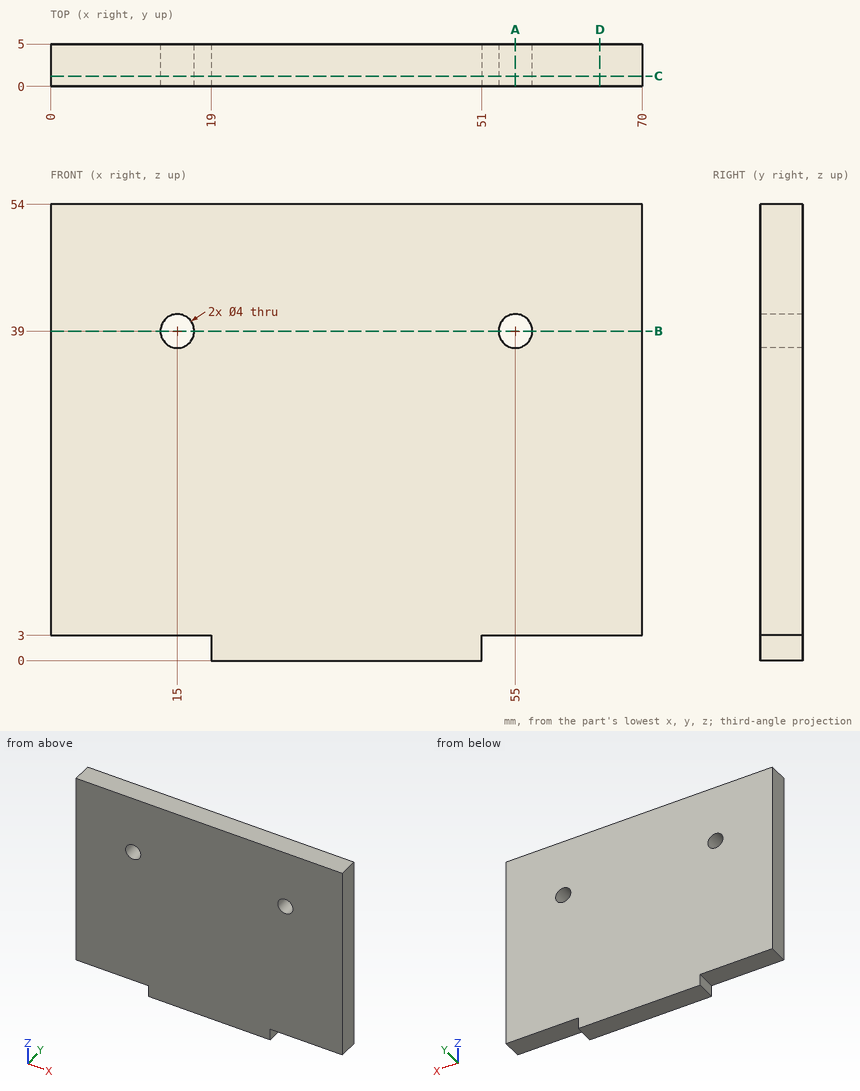
Geometry: see drawing. Coordinates: mm, zero at the bounding-box minimum. Coordinates: 2 decimals unless noted, no trailing zeros. Write each loop counter-clockwise with the first axis right and the second up, starting at its lowest first coordinate (ties: lowest second). Pieces come first, ordered by that corner, then holes. Notation, with made-up numbers: M 81.25,58.5 L 120.25,58.5 A4 ccw 120.25,64.5 Z; hole C 59.25,3 d11. An arc over 180 degrees is marked long. Answer as a JSON object with one key per item and string values.
1. Contact query for flat-ended pins moving along their axis: P1, Ø1.5, axis at x = 63, y = 1.5, coming from the -Z side; P2, Ø0.9, axis at y = 3, z = 2, coming from the -X side; P3, Ø0.9, axis at y = 2.5, z = 1, coming from the +X side. Output: stop coordinate, or through.
Evaluation:
{"P1": "z = 3", "P2": "x = 19", "P3": "x = 51"}
2. Cut plane C-C on y = 1.2. Output: boundary loops of the cut face in (x, z), plus the area to 3 significant figures.
Evaluation:
{"outline": "M 0,3 L 19,3 L 19,0 L 51,0 L 51,3 L 70,3 L 70,54 L 0,54 Z; hole C 15,39 d4; hole C 55,39 d4", "area": "3,640 mm^2"}
3. Cut plane D-D on x = 65. Output: boundary loops of the cut face in (y, z), plus the area to 3 significant figures.
Evaluation:
{"outline": "M 0,3 L 5,3 L 5,54 L 0,54 Z", "area": "255 mm^2"}
4. Ray query, L1, parallel to Z at x = 55, y = 1.8; L2, parallel to X at y = 4.6, z = 38.5. Return the intervals inside material, ascending.
Evaluation:
{"L1": "3 to 37, 41 to 54", "L2": "0 to 13.06, 16.94 to 53.06, 56.94 to 70"}
5. Cut plane B-B on z = 39. Output: boundary loops of the cut face in (x, y).
Evaluation:
{"outline": "M 0,0 L 13,0 L 13,5 L 0,5 Z; M 17,0 L 53,0 L 53,5 L 17,5 Z; M 57,0 L 70,0 L 70,5 L 57,5 Z"}
6. Cut plane A-A on x = 55. Output: boundary loops of the cut face in (y, z), plus the area to 3 significant figures.
Evaluation:
{"outline": "M 0,3 L 5,3 L 5,37 L 0,37 Z; M 0,41 L 5,41 L 5,54 L 0,54 Z", "area": "235 mm^2"}
